```python
from build123d import *

# Parameters (mm, degrees)
BOSS_EXTRUDE1_DEPTH      = 8
BOSS_EXTRUDE2_DEPTH      = 15
BOSS_EXTRUDE4_DEPTH      = 6.3
BOSS_EXTRUDE5_DEPTH      = 6.3
SKETCH7_R                = 1.7
ENL_V_MAT_EXTRU_14_DEPTH = 62.473571557
SKETCH8_W                = 5.8
SKETCH8_H                = 18
BOSS_EXTRU_3_DEPTH       = 0.5
ESQUISSE5_R              = 2.15
ENL_V_MAT_EXTRU_5_DEPTH  = 48.765049984
ESQUISSE9_W              = 28
ESQUISSE9_H              = 5.300857061
ENL_V_MAT_EXTRU_9_DEPTH  = 56.554027757
BOSS_EXTRU_4_DEPTH       = 1
ESQUISSE11_W             = 5.8
ESQUISSE11_H             = 1
BOSS_EXTRU_5_DEPTH       = 1
ESQUISSE14_W             = 6
ESQUISSE14_H             = 5.9
ESQUISSE14_W_2           = 9
BOSS_EXTRU_7_DEPTH       = 23
ESQUISSE15_W             = 0.6
ESQUISSE15_H             = 2
ENL_V_MAT_EXTRU_12_DEPTH = 5.8
ESQUISSE17_W             = 1.2
ESQUISSE17_H             = 5.9
ENL_V_MAT_EXTRU_13_DEPTH = 27
ESQUISSE16_W             = 28
ESQUISSE16_H             = 1
ENL_V_MAT_EXTRU_11_DEPTH = 23
CONG_3_R                 = 4
ENL_V_MAT_EXTRU_15_DEPTH = 2
ENL_V_MAT_EXTRU_16_DEPTH = 2
BOSS_EXTRU_8_DEPTH       = 8


with BuildPart() as part:
    # Sketch1 → Boss-Extrude1 (new body)
    with BuildSketch(Plane(origin=(0, 0, 0), x_dir=(1, 0, 0), z_dir=(0, 1, 0))):
        Polygon((6.3, 0), (6.3, 20.5), (12.5, 20.5), (15.5, 20.5), (21.7, 20.5), (21.7, 0), (28, 0), (36.5, 0), (36.5, 8.5), (28, 8.5), (28, 35), (22, 35), (22, 32), (24, 32), (24, 25), (4, 25), (4, 32), (8, 32), (8, 35), (0, 35), (0, 8.5), (-8.5, 8.5), (-8.5, 0), (0, 0), align=None)
    extrude(amount=BOSS_EXTRUDE1_DEPTH)

    # Sketch2 → Boss-Extrude2 (add)
    with BuildSketch(Plane(origin=(0, 8, 0), x_dir=(1, 0, 0), z_dir=(0, 1, 0))):
        Polygon((8, 35), (8, 32), (4, 32), (4, 25), (24, 25), (24, 32), (22, 32), (22, 35), (28, 35), (28, 20.5), (0, 20.5), (0, 35), align=None)
    extrude(amount=BOSS_EXTRUDE2_DEPTH)

    # Sketch4 → Boss-Extrude4 (add)
    with BuildSketch(Plane.ZY):
        Polygon((-17.5, 23), (-20.5, 23), (-20.5, 8), (-7.5, 8), align=None)
    extrude(amount=-BOSS_EXTRUDE4_DEPTH)

    # Sketch5 → Boss-Extrude5 (add)
    with BuildSketch(Plane(origin=(28, 0, 0), x_dir=(0, 0, -1), z_dir=(1, 0, 0))):
        Polygon((20.5, 8), (7.5, 8), (17.5, 23), (20.5, 23), align=None)
    extrude(amount=-BOSS_EXTRUDE5_DEPTH)

    # Sketch7 → Enlèv. mat.-Extru.14 (cut, through all)
    with BuildSketch(Plane.ZY.offset(8.5)):
        with Locations((-4, 4)):
            Circle(SKETCH7_R)
    extrude(amount=-ENL_V_MAT_EXTRU_14_DEPTH, mode=Mode.SUBTRACT)

    # Sketch8 → Boss.-Extru.3 (add)
    with BuildSketch(Plane(origin=(0, 0, -25), x_dir=(-1, 0, 0), z_dir=(0, 0, -1))):
        with Locations((-14, 9.000007445)):
            Rectangle(SKETCH8_W, SKETCH8_H)
    extrude(amount=BOSS_EXTRU_3_DEPTH)

    # Esquisse5 → Enlèv. mat.-Extru.5 (cut, through all)
    with BuildSketch(Plane.XY.offset(-20.5)):
        with Locations((14.05, 12.4)):
            Circle(ESQUISSE5_R)
    extrude(amount=-ENL_V_MAT_EXTRU_5_DEPTH, mode=Mode.SUBTRACT)

    # Esquisse9 → Enlèv. mat.-Extru.9 (cut, through all)
    with BuildSketch(Plane(origin=(0, 23, 0), x_dir=(1, 0, 0), z_dir=(0, 1, 0))):
        with Locations((14, 34.349571469)):
            Rectangle(ESQUISSE9_W, ESQUISSE9_H)
    extrude(amount=-ENL_V_MAT_EXTRU_9_DEPTH, mode=Mode.SUBTRACT)

    # Esquisse10 → Boss.-Extru.4 (add)
    with BuildSketch(Plane(origin=(0, 0, -25.5), x_dir=(-1, 0, 0), z_dir=(0, 0, -1))):
        Polygon((-16.9, 7.445e-06), (-11.1, 0), (-11.1, 6.800007445), (-16.9, 6.800007445), align=None)
    extrude(amount=BOSS_EXTRU_4_DEPTH)

    # Esquisse11 → Boss.-Extru.5 (add)
    with BuildSketch(Plane(origin=(0, 0, -25), x_dir=(-1, 0, 0), z_dir=(0, 0, -1))):
        with Locations((-14, 18.500007445)):
            Rectangle(ESQUISSE11_W, ESQUISSE11_H)
    extrude(amount=BOSS_EXTRU_5_DEPTH)

    # Esquisse14 → Boss.-Extru.7 (add)
    with BuildSketch(Plane(origin=(0, 23, -10.399142939), x_dir=(-1, 0, 0), z_dir=(0, -1, 0))):
        with Locations((-25, 24.25)):
            Rectangle(ESQUISSE14_W, ESQUISSE14_H)
        with Locations((-4.5, 24.25)):
            Rectangle(ESQUISSE14_W_2, ESQUISSE14_H)
    extrude(amount=BOSS_EXTRU_7_DEPTH)

    # Esquisse15 → Enlèv. mat.-Extru.12 (cut)
    with BuildSketch(Plane(origin=(0, 0, -37.599142939), x_dir=(-1, 0, 0), z_dir=(0, 0, -1))):
        with Locations((-7.5, 17)):
            Rectangle(ESQUISSE15_W, ESQUISSE15_H)
        with Locations((-6.6, 17)):
            Rectangle(ESQUISSE15_W, ESQUISSE15_H)
        with Locations((-5.7, 17)):
            Rectangle(ESQUISSE15_W, ESQUISSE15_H)
        with Locations((-8.4, 17)):
            Rectangle(ESQUISSE15_W, ESQUISSE15_H)
        with Locations((-8.4, 6)):
            Rectangle(ESQUISSE15_W, ESQUISSE15_H)
        with Locations((-0.3, 6)):
            Rectangle(ESQUISSE15_W, ESQUISSE15_H)
        with Locations((-0.3, 17)):
            Rectangle(ESQUISSE15_W, ESQUISSE15_H)
        with Locations((-4.8, 17)):
            Rectangle(ESQUISSE15_W, ESQUISSE15_H)
        with Locations((-3.9, 17)):
            Rectangle(ESQUISSE15_W, ESQUISSE15_H)
        with Locations((-7.5, 6)):
            Rectangle(ESQUISSE15_W, ESQUISSE15_H)
        with Locations((-3, 17)):
            Rectangle(ESQUISSE15_W, ESQUISSE15_H)
        with Locations((-2.1, 17)):
            Rectangle(ESQUISSE15_W, ESQUISSE15_H)
        with Locations((-6.6, 6)):
            Rectangle(ESQUISSE15_W, ESQUISSE15_H)
        with Locations((-1.2, 17)):
            Rectangle(ESQUISSE15_W, ESQUISSE15_H)
        with Locations((-5.7, 6)):
            Rectangle(ESQUISSE15_W, ESQUISSE15_H)
        with Locations((-4.8, 6)):
            Rectangle(ESQUISSE15_W, ESQUISSE15_H)
        with Locations((-3.9, 6)):
            Rectangle(ESQUISSE15_W, ESQUISSE15_H)
        with Locations((-3, 6)):
            Rectangle(ESQUISSE15_W, ESQUISSE15_H)
        with Locations((-2.1, 6)):
            Rectangle(ESQUISSE15_W, ESQUISSE15_H)
        with Locations((-1.2, 6)):
            Rectangle(ESQUISSE15_W, ESQUISSE15_H)
    extrude(amount=-ENL_V_MAT_EXTRU_12_DEPTH, mode=Mode.SUBTRACT)

    # Esquisse17 → Enlèv. mat.-Extru.13 (cut)
    with BuildSketch(Plane(origin=(0, 23, 0), x_dir=(1, 0, 0), z_dir=(0, 1, 0))):
        with Locations((8.407063975, 34.649142939)):
            Rectangle(ESQUISSE17_W, ESQUISSE17_H)
    extrude(amount=-ENL_V_MAT_EXTRU_13_DEPTH, mode=Mode.SUBTRACT)

    # Esquisse16 → Enlèv. mat.-Extru.11 (cut)
    with BuildSketch(Plane(origin=(0, 23, 0), x_dir=(1, 0, 0), z_dir=(0, 1, 0))):
        with Locations((14, 37.099142939)):
            Rectangle(ESQUISSE16_W, ESQUISSE16_H)
    extrude(amount=-ENL_V_MAT_EXTRU_11_DEPTH, mode=Mode.SUBTRACT)

    # Esquisse23 → Enlèvement de matière-Révolution11 (revolve, cut)
    with BuildSketch(Plane(origin=(0, 0, -4), x_dir=(-1, 0, 0), z_dir=(0, 0, -1)), mode=Mode.PRIVATE) as enl_vement_de_mati_re_r_volution11_sk:
        with BuildLine():
            Line((-32.5, 8), (-32.5, 11.823143252))
            Line((-32.5, 11.823143252), (-33.950094463, 11.823143252))
            Line((-33.950094463, 11.823143252), (-37.601757894, 11.944869061))
            Line((-37.601757894, 11.944869061), (-40.320792242, 4))
            Line((-40.320792242, 4), (-36.5, 4))
            ThreePointArc((-36.5, 4), (-35.328427125, 6.828427125), (-32.5, 8))
        make_face()
        with BuildLine():
            Line((8.5, 4), (12.320792242, 4))
            Line((12.320792242, 4), (9.601757894, 11.944869061))
            Line((9.601757894, 11.944869061), (5.950094463, 11.823143252))
            Line((5.950094463, 11.823143252), (4.5, 11.823143252))
            Line((4.5, 11.823143252), (4.5, 8))
            ThreePointArc((4.5, 8), (7.328427125, 6.828427125), (8.5, 4))
        make_face()
    revolve(enl_vement_de_mati_re_r_volution11_sk.sketch.rotate(Axis((36.5, 4, -4), (1, 0, 0)), 90), axis=Axis((36.5, 4, -4), (1, 0, 0)), mode=Mode.SUBTRACT)

    # Congé3
    cong_3_edges = [part.edges().sort_by_distance(p)[0] for p in [
        (27.1, 0, 0),
        (27.1, 8, 0),
        (0.9, 0, 0),
        (0.9, 8, 0),
    ]]
    fillet(cong_3_edges, radius=CONG_3_R - 0.0001)  # a hair under: the kernel refuses the full size

    # Esquisse26 → Enlèv. mat.-Extru.15 (cut)
    with BuildSketch(Plane.ZY.offset(-21.7)):
        Polygon((-0.535898385, 4), (-2.267949192, 7), (-5.732050808, 7), (-7.464101615, 4), (-5.732050808, 1), (-2.267949192, 1), align=None)
    extrude(amount=-ENL_V_MAT_EXTRU_15_DEPTH, mode=Mode.SUBTRACT)

    # Esquisse27 → Enlèv. mat.-Extru.16 (cut)
    with BuildSketch(Plane(origin=(6.3, 0, 0), x_dir=(0, 0, -1), z_dir=(1, 0, 0))):
        Polygon((7.464101615, 4), (5.732050808, 7), (2.267949192, 7), (0.535898385, 4), (2.267949192, 1), (5.732050808, 1), align=None)
    extrude(amount=-ENL_V_MAT_EXTRU_16_DEPTH, mode=Mode.SUBTRACT)

    # Esquisse28 → Boss.-Extru.8 (add)
    with BuildSketch(Plane(origin=(0, 8, 0), x_dir=(1, 0, 0), z_dir=(0, 1, 0))):
        Polygon((28, 8.5), (32.5, 8.5), (28, 14.5), align=None)
        Polygon((-4.5, 8.5), (0, 14.5), (0, 8.5), align=None)
    extrude(amount=-BOSS_EXTRU_8_DEPTH)


solid = part.part
```
Input: part model. Units: mm. Frame: model coordinates. A direction names the side the tool comes from. Give positions to 0.01 mm unless a question says otherwise; leave off trailing zeros. Loops run counter-clockwise (first coordinate to the right, second up) from the corner with the lowest first, then second, coordinate; pieces in that order, holes last. Notation, with made-up numbers: (78.25, 35.5) -> (111.25, 35.5) arc R6 ccw to (111.25, 45.5) -> close; hole circle Ø4 at (64, 88.25). An arc over 180 degrees is marked (long way). Use a Markdown table: item, result.
Q1. Section query D-D, the plane z = -22.5. Return the cut outline in (x, y), plus the area to 3 significant figures.
Entries:
| item | result |
|---|---|
| outline | (0, 0) -> (28, 0) -> (28, 23) -> (0, 23) -> close; hole circle Ø4.3 at (14.05, 12.4) |
| area | 629 mm² |
Q2. First-contact query: P1, Ø3, axis at x = 27, z = -11, coming from the +Y side; P2, Ø1.6, axis at x = 22.5, z = -4, coming from the +Y side; P3, Ø12, axis at x = 15.5, z = -11, coming from the +Y side; P4, Ø6, axis at x = 11.5, y = 10.5, coming from the -Z side. Flat tips, straight axial feed; report the tip coordinate or a pass-through.
Entries:
| item | result |
|---|---|
| P1 | stops at y = 15.5 |
| P2 | stops at y = 8 |
| P3 | passes through |
| P4 | stops at z = -25.5 |
Q3. Section query C-C, the plane y = 13.5. Return the cut outline in (x, z), plus the area to 3 significant figures.
Entries:
| item | result |
|---|---|
| outline | (0, -36.6) -> (7.81, -36.6) -> (7.81, -31.7) -> (4, -31.7) -> (4, -25) -> (11.1, -25) -> (11.1, -25.5) -> (12.2, -25.5) -> (12.2, -20.5) -> (6.3, -20.5) -> (6.3, -11.17) -> (0, -11.17) -> close; (15.9, -25.5) -> (16.9, -25.5) -> (16.9, -25) -> (24, -25) -> (24, -31.7) -> (22, -31.7) -> (22, -36.6) -> (28, -36.6) -> (28, -11.17) -> (21.7, -11.17) -> (21.7, -20.5) -> (15.9, -20.5) -> close |
| area | 349 mm² |
Q4. Ray query, probe 1 along X at (y, z) = (5.5, -26); probe 2 along Y at (x, z) = (1, -4); probe 3 along Y at (x, z) = (14.05, -23.1). Return the intervals inside material, ascending. Write a range as from..to.
Entries:
| item | result |
|---|---|
| probe 1 | x = 0..4, 11.1..16.9, 24..28 |
| probe 2 | y = 0..2.3, 5.7..8 |
| probe 3 | y = 0..10.25, 14.55..23 |
Q5. Access query for faces 1 (the flat face through (4, 11, -28)), 2 (the flat face through (23, 7, -4)), 3 (the flat face through (0.6, 17, -34)), 4 (the flat face through (14, 19, -25.5)), 5 (the flat face through (0.9, 17, -34)). Directions: +Z, -Z, +X, -X, +Y, -Y. A direction counts if a zero-diameter tool reaches every point of the face in a straight line with its end or side. Return the directions, or none.
Entries:
| item | result |
|---|---|
| face 1 | +Y, -Y |
| face 2 | none |
| face 3 | -Z, -X |
| face 4 | -Z, +Y |
| face 5 | -Z |
Q6. Section query A-A, the plane z = -15. Return the cut outline in (x, y).
Entries:
| item | result |
|---|---|
| outline | (0, 0) -> (6.3, 0) -> (6.3, 19.25) -> (0, 19.25) -> close; (21.7, 0) -> (28, 0) -> (28, 19.25) -> (21.7, 19.25) -> close |
Q7. Pull-direction query (Z, two-part tool) for faces 6 (the flat face through (6.3, 9, -15)), 7 (the flat face through (6, 12, -31.699)), 8 (the flat face through (-2.28, 4.06, -11.46)); classes: pulls with the +Z half, pulls with the -Z half, needs draft (parallel to the pull), parting line crosses it, or undercut.
Entries:
| item | result |
|---|---|
| face 6 | needs draft |
| face 7 | undercut |
| face 8 | pulls with the -Z half |
